The figure shows three views and two pictorial views of one solid part (mm, origin at its lowest corner). Answer the questions. Coordinates: 2 decimals unless noted, no trailing zeros. Order: outer loops, then holes, each group sorted by start corner. A loop starts at its lowest first (then second) coordinate and runs counter-clockwise, first axis right, second up. Notation, with made-up numbers: (-17.75, 40.25) - (38.25, 40.25) arc R18 cw to (38.25, 68.25) - close; hole circle Ø11 at (82, 37). An arc over 180 degrees is marked (long way). Use one line per item in the form item = value.
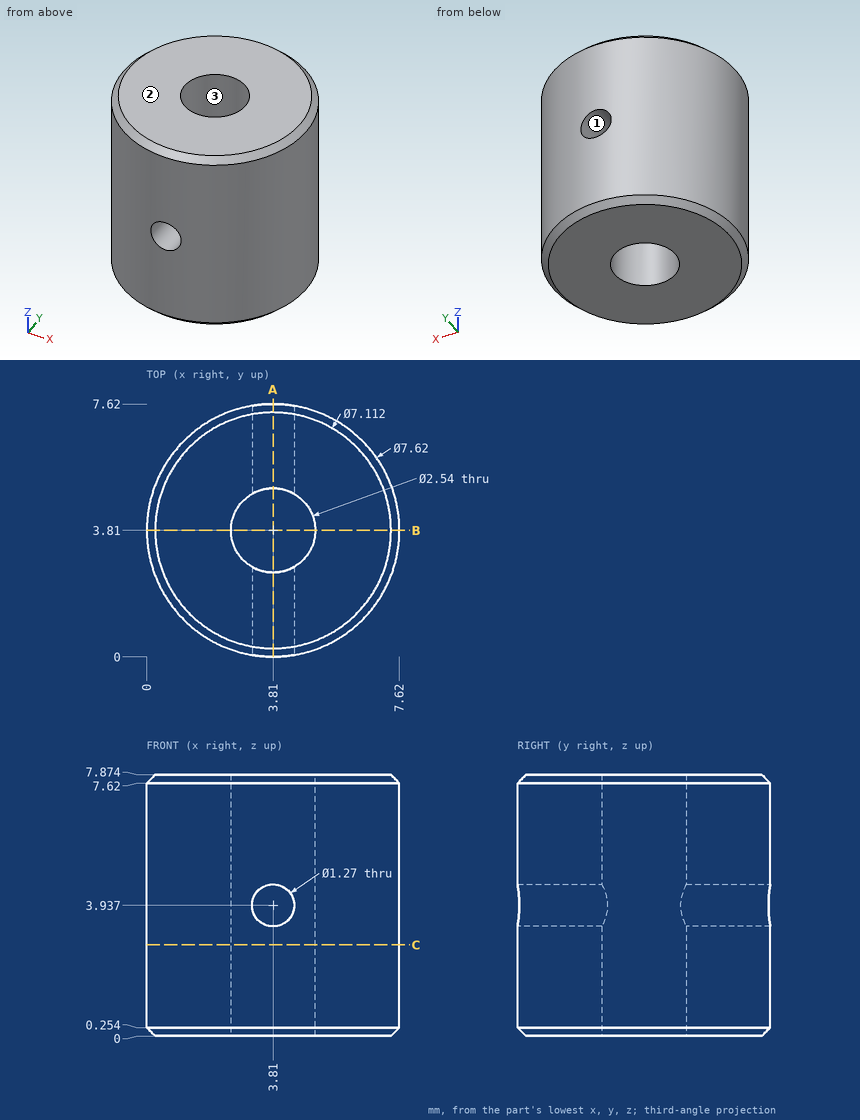
(1) Section C-C, the plane z = 2.75 is taken. Write down the section's boundary in (x, y).
Answer list:
outline = circle Ø7.62 at (3.81, 3.81); hole circle Ø2.54 at (3.81, 3.81)
(2) The mould has two halves that part along Z. Classify the marked faces 1, 2 and 3: +Z half, -Z half, draft (parallel to the pull), parting line (faces both ways), or undercut.
Answer list:
face_1 = undercut
face_2 = +Z half
face_3 = draft
(3) Section A-A, the plane x = 3.81 is taken. Write down the section's boundary in (y, z).
Answer list:
outline = (0, 0.25) - (0.25, 0) - (2.54, 0) - (2.54, 3.3) - (0, 3.3) - close; (0, 4.57) - (2.54, 4.57) - (2.54, 7.87) - (0.25, 7.87) - (0, 7.62) - close; (5.08, 0) - (7.37, 0) - (7.62, 0.25) - (7.62, 3.3) - (5.08, 3.3) - close; (5.08, 4.57) - (7.62, 4.57) - (7.62, 7.62) - (7.37, 7.87) - (5.08, 7.87) - close
(4) Straight lines are drawn through the part: L1, parallel to Z at x = 3.75, y = 2; L2, parallel to Y at x = 4.5, z = 1; L3, parallel to Z at x = 4.25, y = 0.75. For each, find the intervals that lie inside material, in ascending order.
Answer list:
L1 = 0 to 3.3, 4.57 to 7.87
L2 = 0.06 to 2.74, 4.88 to 7.56
L3 = 0 to 3.48, 4.39 to 7.87
(5) Given pin 1 Ø2 at (x, y) = (3.5, 3.5) entering from +Z; pin 2 Ø2 at (x, z) = (7, 2) entering from +Y; pin 3 Ø1.5 at (x, y) = (3.81, 3.81) entering from +Z; pin 4 Ø1.5 at (x, z) = (7, 5) entering from +Y, each flat-ended and moving along its own axis, determine where each tip first touches the part or whether it passes through.
Answer list:
pin_1 = 7.87
pin_2 = 6.93
pin_3 = through
pin_4 = 6.74
(6) Section B-B, the plane y = 3.81 is taken. Write down the section's boundary in (x, z).
Answer list:
outline = (0, 0.25) - (0.25, 0) - (2.54, 0) - (2.54, 7.87) - (0.25, 7.87) - (0, 7.62) - close; (5.08, 0) - (7.37, 0) - (7.62, 0.25) - (7.62, 7.62) - (7.37, 7.87) - (5.08, 7.87) - close
